Work out the finished part from the listing and answer in its coordinate system (mm). A direction names the side the tool comes from. Round coordinates to 2 decimals unless told otherwise and drop trailing zeros. Order: outer loops, then holes, each group sorted by start corner. A loop starts at its lowest first (then second) coordinate and runs counter-clockwise, first axis right, second up. Notation, with made-up numbers: (9.5, -3) - (60.5, -3) arc R22 ccw to (60.5, 16) - close; hole circle Ø2 at (-30.75, -34). An arc over 180 degrees is marked (long way). Use one line per item in the form item = value. Start each with the question number.
Q1. Given P1, Ø0.6, axis at x = 6.5, y = 0.5, coming from the -Z side; P2, Ø2, axis at x = 7.5, z = -11, coming from the -Y side; P3, Ø0.8, axis at x = 5, y = 1, coming from the -Z side; P4, Ø1.2, axis at x = 5.5, z = -5.5, coming from the -Y side, each flat-ended and moving along its own axis, determine where each tip first touches the part or whether it passes through.
Q2. For a pull along Z with two mould halves and no side action, classify faces 4 (the flat face through (0, 3, -6)), 5 (the flat face through (6, 4, -12)), 6 (the flat face through (6, 1, -8.05)) as +Z half, -Z half, draft (parallel to the pull), parting line (faces both ways), or undercut.
Q3. The part is cut by section A-A on y = 1. Determine the outline of the cut face in (x, z).
Q4. The part is cut by section C-C on z = -5.75. Determine the outline of the cut face in (x, y), plus the area to 4 significant figures.
Q5. Which of the six approach directions +Z, -Z, +X, -X, +Y, -Y give full straight-line access (tool end or side, diameter ignored) to faces 1 (the cylindrical face through (0.713, 3.296, -0.752)), 2 (the flat face through (6, 1.2, -11)), 3 (the flat face through (3.95, 1, -6))?
Q6. The part is cut by section D-D on y = 4. Determine the outline of the cut face in (x, z), plus the area to 3 significant figures.
Q7. The part is cut by section B-B on x = 7. Determine the outline of the cut face in (y, z), plus the area to 4 significant figures.
Q8. Find the intervals of material crossed by line 1 (X direction, y = 1.5, z = -4.75); line 2 (Z direction, x = 6, y = 1.75); line 3 (Z direction, x = 6, y = 0.75), in increasing order. Write a range as [from, to].
from build123d import *

# Parameters (mm, degrees)
SKICA1_W                 = 12
SKICA1_H                 = 12
SKICA1_W_2               = 4.1
SKICA1_H_2               = 4.1
P_IDAT_VYSUNUT_M1_DEPTH  = 2.5
SKICA2_W                 = 12
SKICA2_H                 = 12
P_IDAT_VYSUNUT_M2_DEPTH  = 4
ZAOBLIT1_R               = 2.5
SKICA3_W                 = 3
SKICA3_H                 = 1.2
ODEBRAT_VYSUNUT_M1_DEPTH = 13


with BuildPart() as part:
    # Skica1 → Přidat vysunutím1 (new body)
    with BuildSketch(Plane(origin=(0, 0, 0), x_dir=(1, 0, 0), z_dir=(0, 1, 0))):
        with Locations((6, 6)):
            Rectangle(SKICA1_W, SKICA1_H)
        with Locations((6, 6)):
            Rectangle(SKICA1_W_2, SKICA1_H_2, mode=Mode.SUBTRACT)
    extrude(amount=P_IDAT_VYSUNUT_M1_DEPTH)

    # Skica2 → Přidat vysunutím2 (add)
    with BuildSketch(Plane(origin=(0, 2.5, 0), x_dir=(1, 0, 0), z_dir=(0, 1, 0))):
        with Locations((6, 6)):
            Rectangle(SKICA2_W, SKICA2_H)
    extrude(amount=P_IDAT_VYSUNUT_M2_DEPTH)

    # Zaoblit1
    zaoblit1_edges = [part.edges().sort_by_distance(p)[0] for p in [
        (0, 3.25, -12),
        (12, 3.25, -12),
        (12, 3.25, 0),
        (0, 3.25, 0),
    ]]
    fillet(zaoblit1_edges, radius=ZAOBLIT1_R)

    # Skica3 → Odebrat vysunutím1 (cut, through all)
    with BuildSketch(Plane(origin=(12, 0, 0), x_dir=(0, 0, -1), z_dir=(1, 0, 0))):
        with Locations((11, 0.6)):
            Rectangle(SKICA3_W, SKICA3_H)
    extrude(amount=-ODEBRAT_VYSUNUT_M1_DEPTH, mode=Mode.SUBTRACT)


solid = part.part
Found:
q1.P1 = -9.5
q1.P2 = 1.2
q1.P3 = -12
q1.P4 = 2.5
q2.face_4 = draft
q2.face_5 = -Z half
q2.face_6 = undercut
q3.outline = (0, -9.5) - (12, -9.5) - (12, -2.5) arc R2.5 ccw to (9.5, 0) - (2.5, 0) arc R2.5 ccw to (0, -2.5) - close; hole (3.95, -8.05) - (8.05, -8.05) - (8.05, -3.95) - (3.95, -3.95) - close
q4.outline = (0, 0) - (3.95, 0) - (3.95, 2.5) - (8.05, 2.5) - (8.05, 0) - (12, 0) - (12, 6.5) - (0, 6.5) - close
q4.area = 67.75 mm²
q5.face_1 = +Z, -X, +Y, -Y
q5.face_2 = -Z, +X, -X, -Y
q5.face_3 = -Y
q6.outline = (0, -9.5) arc R2.5 ccw to (2.5, -12) - (9.5, -12) arc R2.5 ccw to (12, -9.5) - (12, -2.5) arc R2.5 ccw to (9.5, 0) - (2.5, 0) arc R2.5 ccw to (0, -2.5) - close
q6.area = 139 mm²
q7.outline = (0, -9.5) - (1.2, -9.5) - (1.2, -12) - (6.5, -12) - (6.5, 0) - (0, 0) - (0, -3.95) - (2.5, -3.95) - (2.5, -8.05) - (0, -8.05) - close
q7.area = 64.75 mm²
q8.line_1 = [0, 3.95], [8.05, 12]
q8.line_2 = [-12, -8.05], [-3.95, 0]
q8.line_3 = [-9.5, -8.05], [-3.95, 0]
